```python
from build123d import *

# Parameters (mm, degrees)
RESSALTO_EXTRUS_O1_DEPTH   = 0.1
CORTE_EXTRUS_O1_DEPTH      = 33.458434448
CORTE_EXTRUS_O1_DEPTH_BACK = 33.458434448
ESBO_O2_W                  = 27.4
ESBO_O2_H                  = 19


with BuildPart() as part:
    # Esboço1 → Ressalto-extrusão1 (new body)
    with BuildSketch(Plane.XY):
        with BuildLine():
            Line((-22.158193819, 19.025172981), (-22.158193819, -15.974827019))
            ThreePointArc((-22.158193819, -15.974827019), (-21.279514162, -18.096147362), (-19.158193819, -18.974827019))
            Line((-19.158193819, -18.974827019), (20.841806181, -18.974827019))
            ThreePointArc((20.841806181, -18.974827019), (22.963126525, -18.096147362), (23.841806181, -15.974827019))
            Line((23.841806181, -15.974827019), (23.841806181, 19.025172981))
            ThreePointArc((23.841806181, 19.025172981), (22.963126525, 21.146493325), (20.841806181, 22.025172981))
            Line((20.841806181, 22.025172981), (-19.158193819, 22.025172981))
            ThreePointArc((-19.158193819, 22.025172981), (-21.279514162, 21.146493325), (-22.158193819, 19.025172981))
        make_face()
    extrude(amount=RESSALTO_EXTRUS_O1_DEPTH)

    # Esboço2 → Corte-extrusão1 (cut, two sides: drawn at the far end of the back side and taken through both)
    with BuildSketch(Plane(origin=(0, 0, 0), x_dir=(-1, 0, 0), z_dir=(0, 0, -1)).offset(-CORTE_EXTRUS_O1_DEPTH_BACK)):
        with Locations((-0.841806181, 1.525172981)):
            Rectangle(ESBO_O2_W, ESBO_O2_H)
    extrude(amount=CORTE_EXTRUS_O1_DEPTH + CORTE_EXTRUS_O1_DEPTH_BACK, mode=Mode.SUBTRACT)


solid = part.part
```
Build history of the part. All positions in model axes, mm. Give positions to 0.01 mm unless a question says otherwise; leave off trailing zeros. Loops run counter-clockwise (first coordinate to the right, second up) from the corner with the lowest first, then second, coordinate; pieces in that order, holes last. Notation, with made-up numbers: (77.5, 57.25) - (82.5, 57.25) arc R14 cw to (82.5, 71.25) - close; hole circle Ø5 at (16, -38.75). An arc over 180 degrees is marked (long way). Use a Markdown table: item, result.
(1) Band-saw the part on B-B (x = 3.5). Give the cut face in (y, z).
Taken from the geometry:
| item | result |
|---|---|
| outline | (-18.97, 0) - (-7.97, 0) - (-7.97, 0.1) - (-18.97, 0.1) - close; (11.03, 0) - (22.03, 0) - (22.03, 0.1) - (11.03, 0.1) - close |
(2) Band-saw the part on C-C (z = 0.05). Give the cut face in (x, y), and give its area (3 significant figures).
Taken from the geometry:
| item | result |
|---|---|
| outline | (-22.16, -15.97) arc R3 ccw to (-19.16, -18.97) - (20.84, -18.97) arc R3 ccw to (23.84, -15.97) - (23.84, 19.03) arc R3 ccw to (20.84, 22.03) - (-19.16, 22.03) arc R3 ccw to (-22.16, 19.03) - close; hole (-12.86, -7.97) - (14.54, -7.97) - (14.54, 11.03) - (-12.86, 11.03) - close |
| area | 1,360 mm2 |
(3) Band-saw the part on A-A (y = -1). Give the cut face in (x, z), and give its area (3 significant figures).
Taken from the geometry:
| item | result |
|---|---|
| outline | (-22.16, 0) - (-12.86, 0) - (-12.86, 0.1) - (-22.16, 0.1) - close; (14.54, 0) - (23.84, 0) - (23.84, 0.1) - (14.54, 0.1) - close |
| area | 1.86 mm2 |
(4) Wall check: line 1 along X through (y, z) = (4.5, 0.05); line 2 along Y through (x, z) = (-2, 0.05). Give the ranges that are in metal, low to high.
Taken from the geometry:
| item | result |
|---|---|
| line 1 | -22.16 to -12.86, 14.54 to 23.84 |
| line 2 | -18.97 to -7.97, 11.03 to 22.03 |
